Source: CAD feature listing. Evaluate the final solid. Frame: model axes, mm. Round coordinates to 2 decimals unless told otherwise and drop trailing zeros. Loops run counter-clockwise (first coordinate to the right, second up) from the corner with the lowest first, then second, coordinate; pieces in that order, holes last.
Item 1: Section query B-B on y = 2. Give the number of separate pieces and of enclosed holes in the cut face, then the cut area to 3 significant figures.
Item 2: First-contact query: P1, Ø2, axis at x = -126.63, z = 127.5, coming from the +Y side; P2, Ø4, axis at x = 126.63, z = -127.5, coming from the -Y side. Flat tips, straight axial feed; report the tip coordinate or a pass-through.
Item 3: Section query A-A on x = 32.5. Return loops of the section in (y, z).
Item 4: Ray query, L1, parallel to X at y = 6.5, z = 12.5 (3 decimals); L2, parallel to X at y = 7, z = 127.5 (3 decimals); L3, parallel to Z at x = 0.5, y = 6.75. Return the intervals inside material, ascending.
Item 5: Section query C-C on z = -21.5. Return loops of the section in (x, y) (3 decimals).
```python
from build123d import *

# Parameters (mm, degrees)
SKETCH1_W                      = 273.27
SKETCH1_H                      = 275
BOSS_EXTRUDE1_DEPTH            = 12.7
SKETCH2_W                      = 233.27
SKETCH2_H                      = 235
CUT_EXTRUDE1_DEPTH             = 12.7
M3_CLEARANCE_HOLE1_D           = 3.4
M3_CLEARANCE_HOLE1_CSINK_D     = 3.45
M3_CLEARANCE_HOLE1_CSINK_ANGLE = 90
M3_CLEARANCE_HOLE2_D           = 3.4
M3_CLEARANCE_HOLE2_CSINK_D     = 3.45
M3_CLEARANCE_HOLE2_CSINK_ANGLE = 90


with BuildPart() as part:
    # Sketch1 → Boss-Extrude1 (new body)
    with BuildSketch(Plane(origin=(0, 0, 0), x_dir=(1, 0, 0), z_dir=(0, 1, 0))):
        Rectangle(SKETCH1_W, SKETCH1_H)
    extrude(amount=BOSS_EXTRUDE1_DEPTH)

    # Sketch2 → Cut-Extrude1 (cut)
    with BuildSketch(Plane(origin=(0, 12.7, 0), x_dir=(1, 0, 0), z_dir=(0, 1, 0))):
        Rectangle(SKETCH2_W, SKETCH2_H)
    extrude(amount=-CUT_EXTRUDE1_DEPTH, mode=Mode.SUBTRACT)

    # M3 Clearance Hole1 (through all)
    with Locations(Plane(origin=(0, 12.7, 0), x_dir=(1, 0, 0), z_dir=(0, 1, 0))):
        with Locations((0, 127.5), (-126.635, 127.5), (126.6328, 127.5), (-126.635, 0), (13.3689, -127.5), (113.3689, -127.5), (126.6328, -12.5)):
            CounterSinkHole(M3_CLEARANCE_HOLE1_D / 2, M3_CLEARANCE_HOLE1_CSINK_D / 2, counter_sink_angle=M3_CLEARANCE_HOLE1_CSINK_ANGLE)

    # M3 Clearance Hole2 (through all)
    with Locations(Plane(origin=(0, 12.7, 0), x_dir=(1, 0, 0), z_dir=(0, 1, 0))):
        with Locations((-126.6311, -127.5)):
            CounterSinkHole(M3_CLEARANCE_HOLE2_D / 2, M3_CLEARANCE_HOLE2_CSINK_D / 2, counter_sink_angle=M3_CLEARANCE_HOLE2_CSINK_ANGLE)


solid = part.part
```
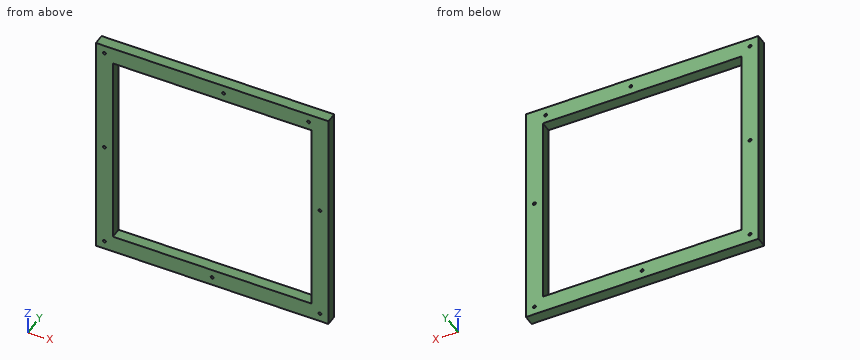
Data:
1. separate pieces: 1
1. enclosed holes: 9
1. area: 20,300 mm2
2. P1: passes through
2. P2: stops at y = 0
3. outline: (0, -137.5) - (12.7, -137.5) - (12.7, -117.5) - (0, -117.5) - close; (0, 117.5) - (12.7, 117.5) - (12.7, 137.5) - (0, 137.5) - close
4. L1: x = -136.635 to -116.635, 116.635 to 124.933, 128.333 to 136.635
4. L2: x = -136.635 to -128.331, -124.931 to 11.669, 15.069 to 111.669, 115.069 to 136.635
4. L3: z = -137.5 to -129.12, -125.88 to -117.5, 117.5 to 137.5
5. outline: (-136.635, 0) - (-116.635, 0) - (-116.635, 12.7) - (-136.635, 12.7) - close; (116.635, 0) - (136.635, 0) - (136.635, 12.7) - (116.635, 12.7) - close
